from build123d import *

# Parameters (mm, degrees)
F1_DEPTH       = 112
F2_W           = 4
F2_H           = 75
F3_DEPTH       = 112.001
F5_DEPTH       = 50
F7_DEPTH       = 50
F9_DEPTH       = 25
F8_R           = 12.5
F10_DEPTH      = 4
F10_DEPTH_BACK = 22
F12_W          = 68
F12_H          = 3
F13_DEPTH      = 56.001
F14_R          = 5
F15_DEPTH      = 25
F16_R          = 4
F17_DEPTH      = 117.001
F18_R          = 4
F19_DEPTH      = 80
F11_R          = 12.5
F20_DEPTH      = 25
F20_DEPTH_BACK = 25
F21_R          = 2.99999


# Not quite as in the source:
# - a fillet or chamfer is up to 0.001 mm smaller than in the source, because OpenCascade refuses the exact size
# - a feature names something its author has since deleted; it is built from what else it names


with BuildPart() as f1:
    # F0 (on Right) → F1 (new body)
    with BuildSketch(Plane.YZ):
        Polygon((-56, 0), (0, 0), (0, 49), (0, 92), (-20, 92), (-20, 37.5714285714), (-56, 17), align=None)
    extrude(amount=F1_DEPTH)

    # F2 (on face) → F3 (cut, through all)
    with BuildSketch(Plane.YZ.offset(112)):
        with Locations((-2, 54.5)):
            Rectangle(F2_W, F2_H)
    extrude(amount=-F3_DEPTH, mode=Mode.SUBTRACT)

    # F4 (on face) → F5 (cut)
    with BuildSketch(Plane.YZ.offset(112)):
        Polygon((-20, 37.5714285714), (-56, 17), (-20, 17), align=None)
    extrude(amount=-F5_DEPTH, mode=Mode.SUBTRACT)

    # F6 (on face) → F7 (cut)
    with BuildSketch(Plane(origin=(0, 0, 0), x_dir=(0, -1, 0), z_dir=(-1, 0, 0))):
        Polygon((20, 17), (56, 17), (20, 37.5714285714), align=None)
    extrude(amount=-F7_DEPTH, mode=Mode.SUBTRACT)

    # F8 (on face) → F9 (cut)
    with BuildSketch(Plane(origin=(0, -4, 0), x_dir=(-1, 0, 0), z_dir=(0, 1, 0))):
        Polygon((-112, 17), (-84, 92), (-112, 92), align=None)
        Polygon((0, 92), (-28, 92), (0, 17), align=None)
    extrude(amount=-F9_DEPTH, mode=Mode.SUBTRACT)

    # F8 (on face) → F10 (join, two sides)
    with BuildSketch(Plane(origin=(0, -4, 0), x_dir=(-1, 0, 0), z_dir=(0, 1, 0))) as f10_sk:
        with BuildLine():
            ThreePointArc((-84, 92), (-56, 64), (-28, 92))
            ThreePointArc((-28, 92), (-56, 120), (-84, 92))
        make_face()
        with Locations((-56, 92)):
            Circle(F8_R, mode=Mode.SUBTRACT)
    extrude(amount=F10_DEPTH)
    extrude(f10_sk.sketch, amount=-F10_DEPTH_BACK)

    # F12 (on face) → F13 (cut, through all)
    with BuildSketch(Plane.XZ.offset(56)):
        with Locations((56, 1.5)):
            Rectangle(F12_W, F12_H)
    extrude(amount=-F13_DEPTH, mode=Mode.SUBTRACT)

    # F14 (on face) → F15 (cut)
    with BuildSketch(Plane.XY.offset(17)):
        with Locations((12, -38)):
            Circle(F14_R)
        with Locations((100, -38)):
            Circle(F14_R)
    extrude(amount=-F15_DEPTH, mode=Mode.SUBTRACT)

    # F16 (on face) → F17 (cut, through all)
    with BuildSketch(Plane(origin=(0, 0, 3), x_dir=(1, 0, 0), z_dir=(0, 0, -1))):
        with Locations((56, 13)):
            Circle(F16_R)
    extrude(amount=-F17_DEPTH, mode=Mode.SUBTRACT)

    # F18 (on face) → F19 (join)
    with BuildSketch(Plane(origin=(0, 0, 3), x_dir=(1, 0, 0), z_dir=(0, 0, -1))):
        with Locations((56, 13)):
            Circle(F18_R)
    extrude(amount=-F19_DEPTH)

    # F11 (on face) → F20 (cut, two sides)
    with BuildSketch(Plane.XZ.offset(20)) as f20_sk:
        with Locations((56, 92)):
            Circle(F11_R)
    extrude(amount=-F20_DEPTH, mode=Mode.SUBTRACT)
    extrude(f20_sk.sketch, amount=F20_DEPTH_BACK, mode=Mode.SUBTRACT)

    # F21 (radius 3 in the source; OpenCascade refuses exactly that, so slightly less here)
    f21_edges = [f1.edges().sort_by_distance(p)[0] for p in [
        (22, -28, 3),
        (90, -28, 3),
    ]]
    fillet(f21_edges, radius=F21_R)


solid = f1.part
The model under review builds one solid part; all positions refer to its coordinate system, in mm. A direction names the side the tool comes from. Give positions to 0.01 mm unless a question says otherwise; leave off trailing zeros. Write each loop counter-clockwise with the first axis right and the second up, starting at its lowest first coordinate (ties: lowest second). Pieces come first, ordered by that corner, then holes.
1. Tool access review of faces 4 (the flat face through (50, -30, 23)), 5 (the flat face through (55.92, -37.75, 27.43)), 6 (the cylindrical face through (22.9, -27.61, 2.14)): name each direction out of +Z, -Z, +X, -X, +Y, -Y from which nothing blocks a thin tool from reaching the whole face with its end or side.
2. Add section C-C, the plane y = -22. Count the separate pieces of the cut face and the enclosed holes in it, plus the area to 3 significant figures.
3. Add section B-B, the plane z = 9. Write out the cut boundary in (x, y).
4. Wall thickness on L1, parallel to Y at x = 12, z = 4.25; L2, parallel to X at y = -36.5, z = 10.5; L3, parallel to Y at x = 56, z = 116.75: over which ranges is each line inside the solid? List them lowest first.
5. Draft analysis for pull direction X (two halves, no side actions). For faces 1 (the cylindrical face through (104.77, -36.5, 8.62)), 2 (the flat face through (14.196, -11.888, 55.025)), 3 (the flat face through (112, -28, 9)), state which applies: +X half, -X half, draft (parallel to the pull), parting line (faces both ways), or undercut.
6. For P1, Ø5, axis at x = 75.5, y = -43.5, coming from the -Z side; P2, Ø6, axis at y = -42, z = 27, coming from the -X side; P3, Ø12, axis at x = 71, z = 55.5, coming from the -Y side; P4, Ø22.5, axis at y = -42.5, z = 26, coming from the +X side, all flat-tipped, find the tip position at first contact; note any pin that passes through.
7. Add section A-A, the plane x = 56. Write out the cut boundary in (y, z), plus the area to 3 significant figures.
Worked answers:
1. face 4: -X, -Y
1. face 5: +X, -X, -Y
1. face 6: -Z, +Y, -Y
2. separate pieces: 2
2. enclosed holes: 1
2. area: 3,910 mm2
3. outline: (0, -56) - (112, -56) - (112, 0) - (0, 0) - close; hole circle Ø10 at (12, -38); hole circle Ø10 at (100, -38)
4. L1: y = -56 to -43, -33 to 0
4. L2: x = 0 to 7.23, 16.77 to 95.23, 104.77 to 112
4. L3: y = -26 to -17, -9 to 0
5. face 1: undercut
5. face 2: -X half
5. face 3: +X half
6. P1: stops at z = 3
6. P2: stops at x = 50
6. P3: stops at y = -20
6. P4: stops at x = 112
7. outline: (-56, 3) - (0, 3) - (0, 17) - (-4, 17) - (-4, 64) - (0, 64) - (0, 79.5) - (-26, 79.5) - (-26, 64) - (-20, 64) - (-20, 37.57) - (-56, 17) - close; (-26, 104.5) - (-17, 104.5) - (-17, 120) - (-26, 120) - close; (-9, 104.5) - (0, 104.5) - (0, 120) - (-9, 120) - close
7. area: 2,590 mm2
